Autodesk Inventor part; units mm, degrees
ref_plane "YZ Plane" through (0, 0, 0) normal (1, 0, 0) x (0, 1, 0)
ref_plane "XZ Plane" through (0, 0, 0) normal (0, 1, 0) x (-1, 0, 0)
ref_plane "XY Plane" through (0, 0, 0) normal (0, 0, 1) x (1, 0, 0)
sketch "Náčrt1" plane through (0, 0, 0) normal (0, 0, 1) x (1, 0, 0)
  line L0 (-8.9, 4.95) -> (-8.9, 14.95)
  line L1 (-8.9, 14.95) -> (-2.15, 14.95)
  line L2 (2.15, 14.95) -> (8.9, 14.95)
  line L3 (8.9, 14.95) -> (8.9, 4.95)
  line L4 (8.9, 4.95) -> (12.9, 4.95)
  line L5 (12.9, 4.95) -> (12.9, -4.95)
  line L6 (12.9, -4.95) -> (8.9, -4.95)
  line L7 (8.9, -4.95) -> (8.9, -14.95)
  line L8 (-8.9, -14.95) -> (-8.9, -4.95)
  line L9 (-12.9, -4.95) -> (-12.9, 4.95)
  line L10 (-12.9, 4.95) -> (-8.9, 4.95)
  line L11 (-8.9, -4.95) -> (-12.9, -4.95)
  arc A0 (-1.9846, 14.5125) -> (1.9846, 14.5125) centre (0, 12.2628) ccw
  arc A1 (-1.9846, 14.5125) -> (-2.15, 14.95) centre (-2.15, 14.7) ccw
  arc A2 (2.15, 14.95) -> (1.9846, 14.5125) centre (2.15, 14.7) ccw
  line L12 (-8.9, -14.95) -> (-2.5458, -14.95)
  arc A3 (2.35, -14.5446) -> (-2.35, -14.5446) centre (0, -12.6798) ccw
  line L13 (2.5458, -14.95) -> (8.9, -14.95)
  arc A4 (-2.5458, -14.95) -> (-2.35, -14.5446) centre (-2.5458, -14.7) ccw
  arc A5 (2.35, -14.5446) -> (2.5458, -14.95) centre (2.5458, -14.7) ccw
  circle A6 centre (5.9, 12.2628) radius 0.5
  point P0 (0, 0)
  point P1 (-1.3338, 14.95)
  point P2 (1.3338, 14.95)
  point P3 (12.9, 0)
  point P4 (-1.9612, -14.95)
  point P5 (1.9612, -14.95)
  dimension "d0" = 9.9
  dimension "d1" = 17.8
  dimension "d2" = 4
  dimension "d4" = 3
  dimension "d5" = 0.25
  dimension "d6" = 3.8
  dimension "d7" = 0.25
  dimension "d8" = 4.7
  dimension "d18" = 1
  dimension "d19" = 3
  dimension "d20" = 10
extrude "Vysunutí1" add sketch "Náčrt1" along normal mid plane 4
properties part number "Spacer"
Build history of the part. All positions in model axes, mm. A direction names the side the tool comes from. Coordinates: 2 decimals unless noted, no trailing zeros. Order: outer loops, then holes, each group sorted by start corner. A loop starts at its lowest first (then second) coordinate and runs counter-clockwise, first axis right, second up. Notation, with made-up numbers: (22, -24.75) -> (78, -24.75) arc R18 cw to (78, -10.75) -> close; hole circle Ø4 at (37, 54.25). An arc over 180 degrees is marked (long way). One line per item, written item: value.
(1) Tool access for faces 1 (the flat face through (8.9, -10, 0)), 2 (the flat face through (-8.9, 10, 0)), 3 (the flat face through (-11, -4.95, 0)): list every direction of +Z, -Z, +X, -X, +Y, -Y with a clear straight run to the whole face (end or side of a thin tool).
Checked values:
face 1: +Z, -Z, +X, -Y
face 2: +Z, -Z, -X, +Y
face 3: +Z, -Z, -X, -Y
(2) Probe line 1 (Y direction, x = -2.5, z = -1.8); line 2 (X direction, y = 7.5, z = 0.3); line 3 (Y direction, x = -9.5, z = 0.2). List the from-to ranges inside material, lowest first. Write a range as [from, to].
Checked values:
line 1: [-14.95, -14.34], [-11.02, 10.6], [13.92, 14.95]
line 2: [-8.9, 8.9]
line 3: [-4.95, 4.95]
(3) Mould opens along Y. For faces 4 (the flat face through (-12.9, 0, 0)), 5 (the flat face through (11, -4.95, 0)), 6 (the cylindrical face through (0.102, 9.265, -0.028)) say: pulls with the +Y half, pulls with the -Y half, needs draft (parallel to the pull), parting line crosses it, or undercut.
Checked values:
face 4: needs draft
face 5: pulls with the -Y half
face 6: undercut
(4) Slice it at A-A, the plane x = 5.9. List the corners of the cut face in (y, z), plus the area to 3 significant figures.
Checked values:
outline: (-14.95, -2) -> (11.76, -2) -> (11.76, 2) -> (-14.95, 2) -> close; (12.76, -2) -> (14.95, -2) -> (14.95, 2) -> (12.76, 2) -> close
area: 116 mm2
(5) Slice it at C-C, the plane z = 1.65. List the corners of the cut face in (x, y), plus the area to 3 significant figures.
Checked values:
outline: (-12.9, -4.95) -> (-8.9, -4.95) -> (-8.9, -14.95) -> (-2.55, -14.95) arc R0.25 ccw to (-2.35, -14.54) arc R3 cw (long way) to (2.35, -14.54) arc R0.25 ccw to (2.55, -14.95) -> (8.9, -14.95) -> (8.9, -4.95) -> (12.9, -4.95) -> (12.9, 4.95) -> (8.9, 4.95) -> (8.9, 14.95) -> (2.15, 14.95) arc R0.25 ccw to (1.98, 14.51) arc R3 cw (long way) to (-1.98, 14.51) arc R0.25 ccw to (-2.15, 14.95) -> (-8.9, 14.95) -> (-8.9, 4.95) -> (-12.9, 4.95) -> close; hole circle Ø1 at (5.9, 12.26)
area: 556 mm2
(6) Slice it at D-D, the plane x = -10.5. List the corners of the cut face in (y, z), plus the area to 3 significant figures.
Checked values:
outline: (-4.95, -2) -> (4.95, -2) -> (4.95, 2) -> (-4.95, 2) -> close
area: 39.6 mm2
(7) Drop flat-ended pins along their axis: pin 1 Ø1 at (x, z) = (1.5, 1.5) entering from -Y; pin 2 Ø1.2 at (y, z) = (-9, -0.5) entering from +X; pin 3 Ø1.2 at (x, z) = (-11.5, -0.5) entering from +Y. Give the stop position or say it passes through.
Checked values:
pin 1: y = -10.44
pin 2: x = 8.9
pin 3: y = 4.95
(8) Slice it at B-B, the plane y = 11.25. List the corners of the cut face in (x, z).
Checked values:
outline: (-8.9, -2) -> (-2.82, -2) -> (-2.82, 2) -> (-8.9, 2) -> close; (2.82, -2) -> (8.9, -2) -> (8.9, 2) -> (2.82, 2) -> close
